Autodesk Fusion 360 part; units mm, degrees
sketch "Sketch1" plane through (0, 0, 0) normal (0, 0, 1) x (1, 0, 0)
  line L0 (-39.5, 22) -> (39.5, 22)
  line L1 (39.5, 22) -> (39.5, -22)
  line L2 (39.5, -22) -> (-39.5, -22)
  line L3 (-39.5, -22) -> (-39.5, 22)
  dimension "d1" = 79
  dimension "d2" = 44
  dimension "d3" = 39.5
  dimension "d4" = 22
extrude "Extrude1" add sketch "Sketch1" along normal blind 4.8
sketch "Sketch2" plane through (0, 0, 4.8) normal (0, 0, 1) x (-1, 0, 0)
  line L0 (39.5, 22) -> (-39.5, 22)
  line L1 (-39.5, 22) -> (-39.5, -22)
  line L2 (-39.5, -22) -> (39.5, -22)
  line L3 (39.5, -22) -> (39.5, 22)
  line L4 (38.3, -20.8) -> (-38.3, -20.8)
  line L5 (-38.3, -20.8) -> (-38.3, 20.8)
  line L6 (-38.3, 20.8) -> (38.3, 20.8)
  line L7 (38.3, 20.8) -> (38.3, -20.8)
  dimension "d7" = 76.6
  dimension "d8" = 41.6
  dimension "d9" = 1.2
  dimension "d10" = 1.2
extrude "Extrude2" cut sketch "Sketch2" against normal blind 3.6 contours L4 L5 L6 L7
sketch "Sketch3" plane through (0, 0, 1.2) normal (0, 0, 1) x (-1, 0, 0)
  line L0 (38.3, 20.8) -> (-38.3, 20.8)
  line L1 (-38.3, 20.8) -> (-38.3, -20.8)
  line L2 (-38.3, -20.8) -> (38.3, -20.8)
  line L3 (38.3, -20.8) -> (38.3, 20.8)
  circle A0 centre (-32.9, -15.4) radius 3.25
  line L4 (39.5, -22) -> (-39.5, -22)
  line L5 (-39.5, -22) -> (-39.5, 22)
  line L6 (39.5, 22) -> (39.5, -22)
  line L7 (-39.5, 22) -> (39.5, 22)
  circle A1 centre (32.9, 15.4) radius 3.25
  line L8 (39.5, 22) -> (39.5, -22)
  line L9 (-39.5, 22) -> (39.5, 22)
  dimension "d13" = 6.5
  dimension "d14" = 6.6
  dimension "d15" = 6.6
  dimension "d29" = 6.5
  dimension "d30" = 6.6
  dimension "d31" = 6.6
sketch "Sketch5" plane through (0, 0, 1.2) normal (0, 0, 1) x (1, 0, 0)
extrude "Extrude4" add sketch "Sketch3" along normal blind 2 contours A1
extrude "Extrude5" cut 1 faces at (-34.1709, -16.2087, 3.2) along direction (0, 0, -1) blind 2
sketch "Sketch6" plane through (0, 0, 0) normal (0, 0, -1) x (1, 0, 0)
  line L0 (39.5, 22) -> (-39.5, 22)
  line L1 (-39.5, 22) -> (-39.5, -22)
  line L2 (-39.5, -22) -> (39.5, -22)
  line L3 (39.5, -22) -> (39.5, 22)
  line L4 (-31.75, 15.4123) -> (-31.75, 18.5877)
  line L5 (-31.75, 18.5877) -> (-34.5, 20.1754)
  line L6 (-34.5, 20.1754) -> (-37.25, 18.5877)
  line L7 (-37.25, 18.5877) -> (-37.25, 15.4123)
  line L8 (-37.25, 15.4123) -> (-34.5, 13.8246)
  line L9 (-34.5, 13.8246) -> (-31.75, 15.4123)
  line L10 (-31.35, 22) -> (-31.35, 13.4246)
  line L11 (-31.35, 13.4246) -> (-39.5, 13.4246)
  point P0 (-34.5, 17)
  dimension "d36" = 2.75
  dimension "d37" = 5
  dimension "d38" = 5
  dimension "d50" = 0.4
  dimension "d51" = 0.4
sketch "Sketch9" plane through (0, 0, 0) normal (0, 0, -1) x (1, 0, 0)
  line L0 (-37.25, -15.4123) -> (-37.25, -18.5877)
  line L1 (-37.25, -18.5877) -> (-34.5, -20.1754)
  line L2 (-34.5, -20.1754) -> (-31.75, -18.5877)
  line L3 (-31.75, -18.5877) -> (-31.75, -15.4123)
  line L4 (-31.75, -15.4123) -> (-34.5, -13.8246)
  line L5 (-34.5, -13.8246) -> (-37.25, -15.4123)
  line L6 (-39.5, 22) -> (-39.5, -22)
  line L7 (-39.5, -22) -> (39.5, -22)
  line L8 (-39.5, -13.0246) -> (-30.95, -13.0246)
  line L9 (-30.95, -13.0246) -> (-30.95, -22)
  point P0 (-34.5, -17)
  dimension "d61" = 2.75
  dimension "d62" = 5
  dimension "d63" = 5
  dimension "d64" = 0.8
  dimension "d65" = 0.8
extrude "Extrude11" add sketch "Sketch9" against normal blind 3.2 contours L0 L1 L2 L3 L4 L5 | L6 L7 L8 L9
extrude "Extrude12" cut sketch "Sketch9" against normal blind 2.4 contours L0 L1 L2 L3 L4 L5
sketch "Sketch10" plane through (0, 0, 3.2) normal (0, 0, 1) x (-1, 0, 0)
  line L0 (38.3, -20.8) -> (38.3, -13.0246)
  line L1 (38.3, -13.0246) -> (30.95, -13.0246)
  line L2 (30.95, -13.0246) -> (30.95, -20.8)
  line L3 (30.95, -20.8) -> (38.3, -20.8)
  circle A0 centre (34.5, -17) radius 1.6
  line L4 (39.5, 22) -> (39.5, -22)
  line L5 (39.5, -22) -> (-39.5, -22)
  dimension "d70" = 3.2
  dimension "d71" = 5
  dimension "d72" = 5
extrude "Extrude13" cut sketch "Sketch10" against normal blind 3.2 contours A0
sketch "Sketch11" plane through (0, 0, 0) normal (0, 0, -1) x (1, 0, 0)
  line L0 (37.25, 15.4123) -> (37.25, 18.5877)
  line L1 (37.25, 18.5877) -> (34.5, 20.1754)
  line L2 (34.5, 20.1754) -> (31.75, 18.5877)
  line L3 (31.75, 18.5877) -> (31.75, 15.4123)
  line L4 (31.75, 15.4123) -> (34.5, 13.8246)
  line L5 (34.5, 13.8246) -> (37.25, 15.4123)
  line L6 (39.5, -22) -> (39.5, 22)
  line L7 (39.5, 22) -> (-39.5, 22)
  line L8 (39.5, 13.0246) -> (30.95, 13.0246)
  line L9 (30.95, 13.0246) -> (30.95, 22)
  point P0 (34.5, 17)
  dimension "d75" = 2.75
  dimension "d76" = 5
  dimension "d77" = 5
  dimension "d78" = 0.8
  dimension "d79" = 0.8
extrude "Extrude14" add sketch "Sketch11" against normal blind 3.2 contours L0 L1 L2 L3 L4 L5 | L6 L7 L8 L9
extrude "Extrude15" cut sketch "Sketch11" against normal blind 2.4 contours L0 L1 L2 L3 L4 L5
sketch "Sketch12" plane through (0, 0, 3.2) normal (0, 0, 1) x (-1, 0, 0)
  line L0 (-38.3, 20.8) -> (-38.3, 13.0246)
  line L1 (-38.3, 13.0246) -> (-30.95, 13.0246)
  line L2 (-30.95, 13.0246) -> (-30.95, 20.8)
  line L3 (-30.95, 20.8) -> (-38.3, 20.8)
  circle A0 centre (-34.5, 17) radius 1.6
  line L4 (-39.5, -22) -> (-39.5, 22)
  line L5 (-39.5, 22) -> (39.5, 22)
  dimension "d84" = 3.2
  dimension "d85" = 5
  dimension "d86" = 5
extrude "Extrude16" cut sketch "Sketch12" against normal blind 3.2 contours A0
sketch "Sketch14" plane through (0, 0, 2.4) normal (0, 0, -1) x (1, 0, 0)
  circle A0 centre (-34.5, -17) radius 1.6
  line L0 (-34.5, -13.8246) -> (-37.25, -15.4123)
  line L1 (-37.25, -15.4123) -> (-37.25, -18.5877)
  line L2 (-37.25, -18.5877) -> (-34.5, -20.1754)
  line L3 (-34.5, -20.1754) -> (-31.75, -18.5877)
  line L4 (-31.75, -18.5877) -> (-31.75, -15.4123)
  line L5 (-31.75, -15.4123) -> (-34.5, -13.8246)
  line L6 (-37.25, -15.4123) -> (-31.75, -15.4123)
  line L7 (-31.75, -18.5877) -> (-37.25, -18.5877)
  line L8 (-36.1, -15.4123) -> (-36.1, -18.5877)
  line L9 (-32.9, -18.5877) -> (-32.9, -15.4123)
sketch "Sketch15" plane through (0, 0, 2.4) normal (0, 0, -1) x (1, 0, 0)
  circle A0 centre (34.5, 17) radius 1.6
  line L0 (34.5, 13.8246) -> (37.25, 15.4123)
  line L1 (37.25, 15.4123) -> (37.25, 18.5877)
  line L2 (37.25, 18.5877) -> (34.5, 20.1754)
  line L3 (34.5, 20.1754) -> (31.75, 18.5877)
  line L4 (31.75, 18.5877) -> (31.75, 15.4123)
  line L5 (31.75, 15.4123) -> (34.5, 13.8246)
  line L6 (31.75, 18.5877) -> (37.25, 18.5877)
  line L7 (37.25, 15.4123) -> (31.75, 15.4123)
  line L8 (32.9, 15.4123) -> (32.9, 18.5877)
  line L9 (36.1, 15.4123) -> (36.1, 18.5877)
extrude "Extrude17" cut sketch "Sketch14" sketch "Sketch15" against normal blind 0.5 contours A0 L7 L9 | A0 L6 L9 | A0 L6 L8 | A0 L7 L8 of sketch 2 contours A0 L7 L9 | A0 L6 L9 | A0 L6 L8 | A0 L7 L8
extrude "Extrude18" cut sketch "Sketch14" sketch "Sketch15" against normal blind 0.2 contours L4 L6 L7 L9 | L1 L6 L7 L8 of sketch 2 contours L1 L6 L7 L9 | L4 L6 L7 L8
extrude "Extrude19" add 4 faces at (35.4826, -19.117, 2.4) (35.4826, -14.883, 2.4) (-33.5174, 14.883, 2.4) (-33.5174, 19.117, 2.4) along direction (0, 0, -1) blind 0.1
sketch "Sketch16" plane through (0, 0, 1.2) normal (0, 0, 1) x (-1, 0, 0)
  line L0 (-30.95, 13.0246) -> (-38.3, 13.0246)
  line L1 (-38.3, 13.0246) -> (-38.3, -20.8)
  line L2 (-38.3, -20.8) -> (30.95, -20.8)
  line L3 (30.95, -20.8) -> (30.95, -13.0246)
  line L4 (30.95, -13.0246) -> (38.3, -13.0246)
  line L5 (38.3, -13.0246) -> (38.3, 20.8)
  line L6 (38.3, 20.8) -> (-30.95, 20.8)
  line L7 (-30.95, 20.8) -> (-30.95, 13.0246)
  line L8 (-30.95, -20.8) -> (-38.3, -20.8)
  line L9 (-38.3, -20.8) -> (-38.3, -13.025)
  line L10 (-38.3, -13.025) -> (-30.95, -13.025)
  line L11 (-30.95, -13.025) -> (-30.95, -20.8)
  line L12 (38.3, 20.8) -> (38.3, 13.025)
  line L13 (38.3, 13.025) -> (30.95, 13.025)
  line L14 (30.95, 20.8) -> (38.3, 20.8)
  line L15 (30.95, 13.025) -> (30.95, 20.8)
  dimension "d95" = 7.35
  dimension "d96" = 7.775
  dimension "d97" = 7.35
  dimension "d98" = 7.775
extrude "Extrude20" add sketch "Sketch16" along normal blind 2 contours L1 L2 L8 L9 L10 L11 | L5 L6 L12 L13 L14 L15
extrude "Extrude21" add 1 faces at (-13.1667, -7.3333, 0) along direction (0, 0, -1) blind 0.3
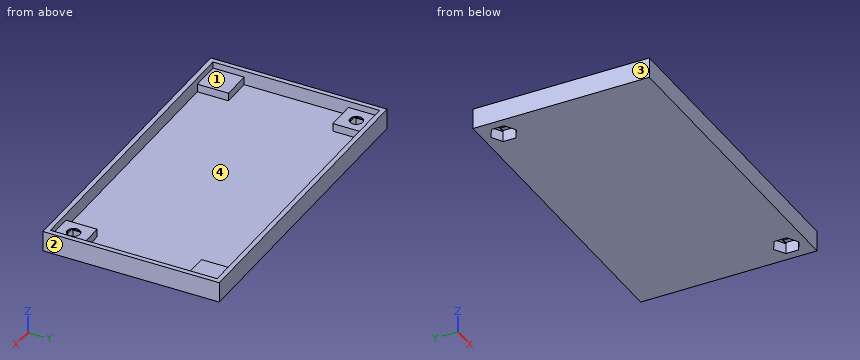
Work out the finished part from the listing and answer in its coordinate system (mm). Face numbers are marked on the shaded views. A direction names the side the tool comes from. Round coordinates to 2 decimals unless told otherwise and drop trailing zeros. Loops run counter-clockwise (first coordinate to the right, second up) from the corner with the lowest first, then second, coordinate; pieces in that order, holes last.
(1) The part is cut by section B-B, the plane y = -11.5. Give the vertices of the cut face in (x, z).
Computed values:
outline: (-39.5, -0.3) - (39.5, -0.3) - (39.5, 4.8) - (38.3, 4.8) - (38.3, 1.2) - (-38.3, 1.2) - (-38.3, 4.8) - (-39.5, 4.8) - close
(2) The part is cut by section A-A, the plane x = 26.5. Give the vertices of the cut face in (y, z).
Computed values:
outline: (-22, -0.3) - (22, -0.3) - (22, 4.8) - (20.8, 4.8) - (20.8, 1.2) - (-20.8, 1.2) - (-20.8, 4.8) - (-22, 4.8) - close
(3) The mould has two halves that part along Y. Classify the marked faces 1 and 2: pulls with the +Y half, pulls with the -Y half, needs draft (parallel to the pull), parting line crosses it, or undercut.
Computed values:
face 1: undercut
face 2: needs draft
(4) Each of these flat-tipped pins is pushed along its axis until it touches: P1, Ø0.9, axis at x = -32.5, y = 16.5, coming from the -Z side; P2, Ø6, axis at x = 26.5, y = 7.5, coming from the +Z side; P3, Ø5, axis at x = 34.5, y = -17, coming from the -Z side. Where does it stop, or does it pass through?
Computed values:
P1: stops at z = 2.6
P2: stops at z = 1.2
P3: stops at z = 2.3
(5) Find the intervals of material crossed by L1, parallel to Y at x = 34.5, z = 2.5 (3 decimals); L2, parallel to X at y = -17, z = 2.55; L3, parallel to Y at x = -34.5, z = 2.9 (3 decimals), in increasing order.
Computed values:
L1: y = -22 to -18.6, -15.4 to -13.025, 13.025 to 22
L2: x = -39.5 to -30.95, 30.95 to 31.75, 37.25 to 39.5
L3: y = -22 to -13.025, 13.025 to 15.4, 18.6 to 22
(6) For the marked faces 3 and 4, determine the directions among +Z, -Z, +X, -X, +Y, -Y from which every point of the face is accessible in a straight line to the end or side of a thin tool.
Computed values:
face 3: +Z, -Z, -X, +Y, -Y
face 4: +Z
